```python
from build123d import *

# Parameters (mm, degrees)
SKETCH_1_R             = 5
SKETCH_1_R_2           = 27
SM_BASE_FLANGE_1_DEPTH = 6
SKETCH_6_R             = 3.5
SKETCH_6_R_2           = 3
CUT_EXTRUDE_1_DEPTH    = 106.298498587
CHAMFER_1_SIZE         = 3


# Sheet-metal steps are written as plain solids
with BuildPart() as part:
    # Sketch 1 → Базовая кромка1 (new body)
    with BuildSketch(Plane.XY):
        with BuildLine():
            Line((74.336309448, -66.888811454), (74.336309448, 66.888811454))
            ThreePointArc((74.336309448, 66.888811454), (70.710678119, 70.710678119), (66.888811454, 74.336309448))
            Line((66.888811454, 74.336309448), (-66.888811454, 74.336309448))
            ThreePointArc((-66.888811454, 74.336309448), (-70.710678119, 70.710678119), (-74.336309448, 66.888811454))
            Line((-74.336309448, 66.888811454), (-74.336309448, -66.888811454))
            ThreePointArc((-74.336309448, -66.888811454), (-70.710678119, -70.710678119), (-66.888811454, -74.336309448))
            Line((-66.888811454, -74.336309448), (66.888811454, -74.336309448))
            ThreePointArc((66.888811454, -74.336309448), (70.710678119, -70.710678119), (74.336309448, -66.888811454))
        make_face()
        with Locations((-58.336309448, -58.336309448)):
            Circle(SKETCH_1_R, mode=Mode.SUBTRACT)
        with Locations((-58.336309448, 58.336309448)):
            Circle(SKETCH_1_R, mode=Mode.SUBTRACT)
        with Locations((58.336309448, 58.336309448)):
            Circle(SKETCH_1_R, mode=Mode.SUBTRACT)
        with Locations((58.336309448, -58.336309448)):
            Circle(SKETCH_1_R, mode=Mode.SUBTRACT)
        Circle(SKETCH_1_R_2, mode=Mode.SUBTRACT)
    extrude(amount=-SM_BASE_FLANGE_1_DEPTH)

    # Эскиз6 → Вырез-Вытянуть1 (cut, through all)
    with BuildSketch(Plane.XY):
        with Locations((-32.454521271, 67.836309448)):
            Circle(SKETCH_6_R)
        with Locations((-42.621905135, 14.435137777)):
            Circle(SKETCH_6_R_2)
        with Locations((-14.435137777, -42.621905135)):
            Circle(SKETCH_6_R_2)
        with Locations((42.621905135, -14.435137777)):
            Circle(SKETCH_6_R_2)
        with Locations((66.996590711, 34.154321301)):
            Circle(SKETCH_6_R)
    extrude(amount=-CUT_EXTRUDE_1_DEPTH, mode=Mode.SUBTRACT)

    # Фаска1
    chamfer_1_edges = [part.edges().sort_by_distance(p)[0] for p in [
        (-35.954521271, 67.836309448, 0),
        (-45.621905135, 14.435137777, 0),
        (-17.435137777, -42.621905135, 0),
        (39.621905135, -14.435137777, 0),
        (63.496590711, 34.154321301, 0),
    ]]
    chamfer(chamfer_1_edges, length=CHAMFER_1_SIZE - 0.0001)  # a hair under: the kernel refuses the full size


solid = part.part
```
For this review, take the finished solid that the model builds, in its own axes (mm). Give positions to 0.01 mm unless a question says otherwise; leave off trailing zeros. Loops run counter-clockwise (first coordinate to the right, second up) from the corner with the lowest first, then second, coordinate; pieces in that order, holes last. Notation, with made-up numbers: M 48,-16 L 85,-16 A15 cw 85,-12 Z; hole C 77,33.25 d7. An arc over 180 degrees is marked long. One line per item, written item: value. Start each with the question number.
Q1. For L1, parallel to Y at x = 58, z = -3; L2, parallel to X at y = 61, z = -2.75; L3, parallel to Y at x = -62, z = -3.75, list the stretches that pass through material, from the lowest coordinate up.
Q2. Draft analysis for pull direction X (two halves, no side actions). For faces 1 (the face through (-70.66, 70.76, -2.96)), 2 (the face through (-30.84, 64.73, -4.48)), 3 (the face through (1, 74.336, -3)), state which applies: released by +X, released by -X, zero draft, split by the parting line, or undercut.
Q3. Add section C-C (z = -1.25). Count the separate pieces of the cut face and the enclosed holes in it, and give its area (3 significant figures).
Q4. Clearance check with flat-ended pins moving along their axes: pin 1 Ø5 at (x, y) = (20, 12.5) entering from -Z; pin 2 Ø8 at (x, y) = (-42.62, 14.44) entering from +Z; pin 3 Ø9.5 at (x, y) = (42.62, -14.44) entering from +Z. State where each tip first meets the part, or that it passes through.
Q5. Add section D-D (x = -61). Give the boundary of the cut face in (y, z), and give its area (3 significant figures).
Q6. Add section A-A (x = 0). Give the boundary of the cut face in (y, z).
Reply:
1. L1: -74.34 to -63.32, -53.35 to 53.35, 63.32 to 74.34
1. L2: -74.34 to -62.57, -54.1 to 54.1, 62.57 to 74.34
1. L3: -74.34 to -61.74, -54.93 to 54.93, 61.74 to 74.34
2. face 1: released by -X
2. face 2: undercut
2. face 3: zero draft
3. separate pieces: 1
3. enclosed holes: 10
3. area: 19,000 mm²
4. pin 1: through
4. pin 2: z = -1.99
4. pin 3: z = -1.24
5. outline: M -74.34,-6 L -62.57,-6 L -62.57,0 L -74.34,0 Z; M -54.1,-6 L 54.1,-6 L 54.1,0 L -54.1,0 Z; M 62.57,-6 L 74.34,-6 L 74.34,0 L 62.57,0 Z
5. area: 790 mm²
6. outline: M -74.34,-6 L -27,-6 L -27,0 L -74.34,0 Z; M 27,-6 L 74.34,-6 L 74.34,0 L 27,0 Z
